Check sheet for the modelled part. Datum: model origin and axes. Units: mm. A direction names the side the tool comes from. Give positions to 0.01 mm unless a question says otherwise; leave off trailing zeros. Loops run counter-clockwise (first coordinate to the right, second up) from the corner with the lowest first, then second, coordinate; pieces in that order, holes last. Notation, with made-up numbers: (58.5, -22.5) - (71.5, -22.5) arc R15 ccw to (71.5, 5.5) - close; hole circle Ø5 at (-26.5, 64). An arc over 180 degrees is marked (long way). Use one line per item in the form item = value.
from build123d import *

# Parameters (mm, degrees)
BASE_EXTRUDE_DEPTH = 3


with BuildPart() as part:
    # Sketch1 → Base-Extrude (new body)
    with BuildSketch(Plane.XY):
        with BuildLine():
            Line((1123.682056814, 62.226353312), (1123.217824039, 92.222761229))
            ThreePointArc((1123.217824039, 92.222761229), (1131.93888948, 94.9852284), (1138.016482209, 101.822704098))
            Line((1138.016482209, 101.822704098), (1140.223428748, 100.122354582))
            Line((1140.223428748, 100.122354582), (1149.427763829, 81.453359638))
            Line((1149.427763829, 81.453359638), (1142.423370566, 78.994416072))
            Line((1142.423370566, 78.994416072), (1143.41708769, 76.163775459))
            Line((1143.41708769, 76.163775459), (1150.764055432, 78.742982306))
            Line((1150.764055432, 78.742982306), (1157.735111853, 64.603708156))
            Line((1157.735111853, 64.603708156), (1151.41486057, 64.603708156))
            Line((1151.41486057, 64.603708156), (1151.41486057, 61.603708156))
            Line((1151.41486057, 61.603708156), (1157.735111853, 61.603708156))
            Line((1157.735111853, 61.603708156), (1148.914752181, 48.53787652))
            Line((1148.914752181, 48.53787652), (1141.376892152, 51.634018924))
            Line((1141.376892152, 51.634018924), (1140.237061373, 48.858989953))
            Line((1140.237061373, 48.858989953), (1147.661839843, 45.809295294))
            Line((1147.661839843, 45.809295294), (1140.993007118, 38.529613243))
            Line((1140.993007118, 38.529613243), (1135.426293127, 44.164590139))
            Line((1135.426293127, 44.164590139), (1133.292085124, 42.056236232))
            Line((1133.292085124, 42.056236232), (1139.086791645, 36.190471003))
            Line((1139.086791645, 36.190471003), (1125.452564162, 34.76659158))
            Line((1125.452564162, 34.76659158), (1115.659628086, 46.499294412))
            Line((1115.659628086, 46.499294412), (1115.559210016, 76.887215732))
            ThreePointArc((1115.559210016, 76.887215732), (1116.142650811, 78.305699753), (1117.559199096, 78.893824774))
            Line((1117.559199096, 78.893824774), (1118.454460183, 78.893824774))
            ThreePointArc((1118.454460183, 78.893824774), (1119.857689012, 78.318938401), (1120.454220711, 76.924773625))
            Line((1120.454220711, 76.924773625), (1120.682416022, 62.179930034))
            Line((1120.682416022, 62.179930034), (1123.682056814, 62.226353312))
        make_face()
    extrude(amount=BASE_EXTRUDE_DEPTH)


solid = part.part
Item 1: Section check C-C on y = 72. Record the boundary of the cut face in (x, z).
Answer block:
outline = (1115.58, 0) - (1120.53, 0) - (1120.53, 3) - (1115.58, 3) - close; (1123.53, 0) - (1154.09, 0) - (1154.09, 3) - (1123.53, 3) - close
Item 2: Section check A-A on x = 1147. Record the boundary of the cut face in (y, z).
Answer block:
outline = (45.09, 0) - (46.08, 0) - (46.08, 3) - (45.09, 3) - close; (49.32, 0) - (77.42, 0) - (77.42, 3) - (49.32, 3) - close; (80.6, 0) - (86.38, 0) - (86.38, 3) - (80.6, 3) - close
Item 3: Thickness scan on L1, parallel to Y at x = 1144, z = 2; L2, parallel to Y at x = 1145, z = 0.4; L3, parallel to X at y = 49, z = 0.5. Record the ranges inside material, lowest first.
Answer block:
L1 = 41.81 to 47.31, 50.56 to 76.37, 79.55 to 92.46
L2 = 42.9 to 46.9, 50.15 to 76.72, 79.9 to 90.43
L3 = 1115.65 to 1140.29, 1147.79 to 1149.23
Item 4: Access from +Z, -Z, +X, -X, +Y, -Y to the whole of each face (thin tool, end or side, straight path). Record for faces 1 (the face through (1155, 64.604, 1)), 2 (the face through (1119.842, 78.334, 1.479)), 3 (the face through (1145.199, 50.064, 1.479)).
Answer block:
face_1 = +Z, -Z, +X
face_2 = +Z, -Z, +Y
face_3 = +Z, -Z
Item 5: Section check B-B on z = 1.9. Record the boundary of the cut face in (x, y), then the cut area to 3 significant figures.
Answer block:
outline = (1115.56, 76.89) - (1115.66, 46.5) - (1125.45, 34.77) - (1139.09, 36.19) - (1133.29, 42.06) - (1135.43, 44.16) - (1140.99, 38.53) - (1147.66, 45.81) - (1140.24, 48.86) - (1141.38, 51.63) - (1148.91, 48.54) - (1157.74, 61.6) - (1151.41, 61.6) - (1151.41, 64.6) - (1157.74, 64.6) - (1150.76, 78.74) - (1143.42, 76.16) - (1142.42, 78.99) - (1149.43, 81.45) - (1140.22, 100.12) - (1138.02, 101.82) arc R17.23 cw to (1123.22, 92.22) - (1123.68, 62.23) - (1120.68, 62.18) - (1120.45, 76.92) arc R2 ccw to (1118.45, 78.89) - (1117.56, 78.89) arc R2 ccw to start
area = 1,750 mm2
Item 6: Section check D-D on x = 1153. Record the boundary of the cut face in (y, z).
Answer block:
outline = (54.59, 0) - (61.6, 0) - (61.6, 3) - (54.59, 3) - close; (64.6, 0) - (74.21, 0) - (74.21, 3) - (64.6, 3) - close
Item 7: Gauge pin test, flat ends, axial feed: P1, Ø0.9, axis at x = 1156, z = 1.5, coming from the +Y side; P2, Ø1.5, axis at y = 50, z = 1.5, coming from the +X side. Record the tip position at first contact, or that the pin passes through.
Answer block:
P1 = 69.04
P2 = 1150.41
Item 8: Mould release check, pull along X, two halves, no side actions. Record for faces 4 (the face through (1145.97, 80.24, 1.48)), 5 (the face through (1147.039, 77.435, 1.479)), 6 (the face through (1155, 61.604, 1)): released by +X, released by -X, zero draft, split by the parting line, or undercut.
Answer block:
face_4 = released by +X
face_5 = undercut
face_6 = zero draft
